Model file for the job. Use its own axes, mm. Coordinates: 2 decimals unless noted, no trailing zeros. Loops run counter-clockwise (first coordinate to the right, second up) from the corner with the lowest first, then second, coordinate; pieces in that order, holes last. Notation, with made-up numbers: (-14, 21.25) -> (13, 21.25) arc R10 ccw to (13, 32.25) -> close; hole circle Ø11 at (11, 3). An arc over 180 degrees is marked (long way). Use one line per item in the form item = value.
Autodesk Inventor part; units mm, degrees
ref_plane "YZ Plane" through (0, 0, 0) normal (1, 0, 0) x (0, 1, 0)
ref_plane "XZ Plane" through (0, 0, 0) normal (0, 1, 0) x (-1, 0, 0)
ref_plane "XY Plane" through (0, 0, 0) normal (0, 0, 1) x (1, 0, 0)
sketch "Boceto1" plane through (0, 0, 0) normal (0, 0, 1) x (1, 0, 0)
  line L0 (-18.4596, -13.534) -> (-18.4596, -15.934)
  line L1 (-18.4596, -15.934) -> (-19.8596, -15.934)
  line L2 (-19.8596, -15.934) -> (-19.8596, -13.934)
  line L3 (-19.8596, -13.934) -> (-21.3596, -13.934)
  line L4 (-21.3596, -13.934) -> (-21.3596, -21.934)
  line L5 (-21.3596, -21.934) -> (-19.8596, -21.934)
  line L6 (-19.8596, -21.934) -> (-19.8596, -19.934)
  line L7 (-19.8596, -19.934) -> (-18.4596, -19.934)
  line L8 (-18.4596, -19.934) -> (-18.4596, -22.334)
  line L9 (-18.4596, -13.534) -> (-16.4596, -13.534)
  line L10 (-16.4596, -13.534) -> (-16.4596, -22.334)
  line L11 (-16.4596, -22.334) -> (-18.4596, -22.334)
  point P0 (-26.2596, -17.734)
  point P1 (-21.3596, -17.934)
  dimension "d28" = 1.4
  dimension "d30" = 1.4
  dimension "d34" = 8
  dimension "d35" = 2
  dimension "d36" = 4
  dimension "d37" = 1.5
  dimension "d64" = 8.8
  dimension "d65" = 2
extrude "Extrusión1" add sketch "Boceto1" against normal blind 1129
ref_plane "Plano de trabajo2" through (0, 0, -564.5) normal (0, 0, -1) x (-1, 0, 0)
sketch "Boceto3" plane through (-16.4596, -22.334, 0) normal (1, 0, 0) x (0, 0, -1)
  line L0 (0, 0) -> (0, 8.8)
  line L1 (0, 0) -> (1129, 0)
  line L2 (1129, 8.8) -> (1129, 0)
  line L3 (0, 8.8) -> (1129, 8.8)
  line L4 (0, 0) -> (8.8, 8.8)
  line L5 (8.8, 8.8) -> (0, 8.8)
  line L6 (0, 0) -> (0, 8.8)
  point P0 (0, 22.334)
  dimension "d69" = 45
extrude "Extrusión2" cut sketch "Boceto3" against normal blind 692.2 contours L0 L3 L4
mirror "Simetría2" about plane through (0, 0, -564.5) normal (0, 0, -1) of "Extrusión2"
properties part number "JUNTA DE FELPA 1128 mm" material "Caucho"
Q1. Wall check: line 1 along X through (y, z) = (-14.75, -516); line 2 along Y through (x, z) = (-18.65, -149); line 3 along Y through (x, z) = (-19.9, -985). Give the ranges that are in metal, low to high.
Result:
line_1 = -21.36 to -19.86, -18.46 to -16.46
line_2 = -19.93 to -15.93
line_3 = -21.93 to -13.93
Q2. Pin check, flat tips, straight feed: pin 1 Ø0.8 at (x, z) = (-21, -420.5) entering from -Y; pin 2 Ø1.5 at (x, z) = (-19, -668) entering from +Y; pin 3 Ø1.5 at (x, y) = (-20, -21) entering from +Z; pin 4 Ø0.8 at (x, z) = (-20.5, -740) entering from +Y. Stop position of each tip, or through.
Result:
pin_1 = -21.93
pin_2 = -13.53
pin_3 = -0.58
pin_4 = -13.93
Q3. Band-saw the part on A-A, the plane z = -487.5. Write the cut outline in (x, y), and give its area (3 significant figures).
Result:
outline = (-21.36, -21.93) -> (-19.86, -21.93) -> (-19.86, -19.93) -> (-18.46, -19.93) -> (-18.46, -22.33) -> (-16.46, -22.33) -> (-16.46, -13.53) -> (-18.46, -13.53) -> (-18.46, -15.93) -> (-19.86, -15.93) -> (-19.86, -13.93) -> (-21.36, -13.93) -> close
area = 35.2 mm2
